from build123d import *

# Parameters (mm, degrees)
EXTRUDE1_DEPTH     = 16.75
SKETCH3_R          = 1.1
CUT_EXTRUDE1_DEPTH = 20.798295381
SKETCH5_R          = 4.1
CUT_EXTRUDE2_DEPTH = 24


with BuildPart() as part:
    # Sketch1 → Extrude1 (new body)
    with BuildSketch(Plane.XY):
        with BuildLine():
            Line((-4.6, -8.312039461), (-4.6, 8.312039461))
            ThreePointArc((-4.6, 8.312039461), (0, 9.5), (4.6, 8.312039461))
            Line((4.6, 8.312039461), (4.6, -8.312039461))
            ThreePointArc((4.6, -8.312039461), (0, -9.5), (-4.6, -8.312039461))
        make_face()
    extrude(amount=EXTRUDE1_DEPTH)

    # Sketch3 → Cut-Extrude1 (cut, through all)
    with BuildSketch(Plane.XY.offset(16.75)):
        with Locations((0, 6.715)):
            Circle(SKETCH3_R)
        with Locations(Location((0, -6.715, 0), (0, 0, 180))):
            Circle(SKETCH3_R)
    extrude(amount=-CUT_EXTRUDE1_DEPTH, mode=Mode.SUBTRACT)

    # Sketch5 → Cut-Extrude2 (cut)
    with BuildSketch(Plane(origin=(0, 0, 0), x_dir=(-1, 0, 0), z_dir=(0, 0, -1))):
        Circle(SKETCH5_R)
    extrude(amount=-CUT_EXTRUDE2_DEPTH, mode=Mode.SUBTRACT)


solid = part.part
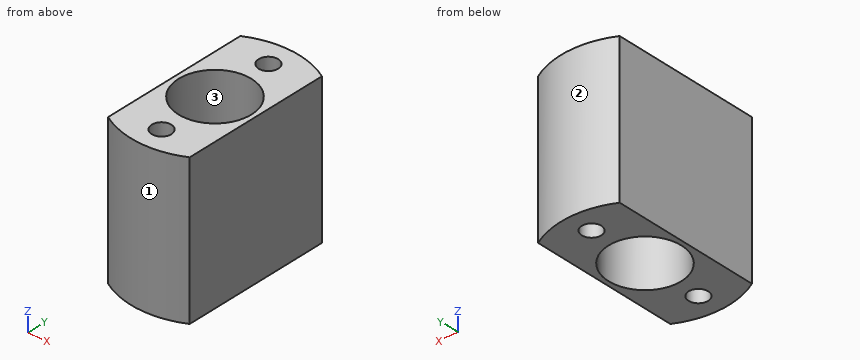
Can you work these out from the model? Positions are in its coordinate system, mm. Face numbers are marked on the shaded views. Coordinates: 2 decimals unless noted, no trailing zeros. Order: outer loops, then holes, each group sorted by start corner. A loop starts at its lowest first (then second) coordinate and runs counter-clockwise, first axis right, second up. Notation, with made-up numbers: M 88.25,-7.75 L 102.25,-7.75 A18 ccw 102.25,17.25 Z; hole C -24,76 d8. An arc over 180 degrees is marked long. Answer as CSV lines item,"result".
(1) Suppose I cut it at D-D on z = 11.5. Please give me the cut outline in (x, y) (3 decimals), plus the area to 3 significant figures.
Geometry check:
outline,"M -4.6,-8.312 A9.5 ccw 4.6,-8.312 L 4.6,8.312 A9.5 ccw -4.6,8.312 Z; hole C 0,0 d8.2; hole C 0,-6.715 d2.2; hole C 0,6.715 d2.2"
area,"107 mm^2"
(2) Suppose I cut it at B-B on x = 0. Please give me the cut outline in (y, z) (3 decimals).
Geometry check:
outline,"M -9.5,0 L -7.815,0 L -7.815,16.75 L -9.5,16.75 Z; M -5.615,0 L -4.1,0 L -4.1,16.75 L -5.615,16.75 Z; M 4.1,0 L 5.615,0 L 5.615,16.75 L 4.1,16.75 Z; M 7.815,0 L 9.5,0 L 9.5,16.75 L 7.815,16.75 Z"
(3) Suppose I cut it at A-A on y = 0. Please give me the cut outline in (x, z), plus the area to 4 significant figures.
Geometry check:
outline,"M -4.6,0 L -4.1,0 L -4.1,16.75 L -4.6,16.75 Z; M 4.1,0 L 4.6,0 L 4.6,16.75 L 4.1,16.75 Z"
area,"16.75 mm^2"
(4) If we mould it in two halves opening along Y, with no side actions, what happens to the marked faces 1, 2 and 3? For each: released by +Y, released by -Y, zero draft, split by the parting line, or undercut.
Geometry check:
face 1,"released by -Y"
face 2,"released by +Y"
face 3,"undercut"
(5) Please list where these lines run through material, in increasing order: L1, parallel to Y at x = 1.25, z = 15.25; L2, parallel to X at y = -2, z = 14.5; L3, parallel to X at y = -6, z = 8.5.
Geometry check:
L1,"-9.42 to -3.9, 3.9 to 9.42"
L2,"-4.6 to -3.58, 3.58 to 4.6"
L3,"-4.6 to -0.84, 0.84 to 4.6"
(6) Suppose I cut it at C-C on x = 1.5. Please give me the cut outline in (y, z).
Geometry check:
outline,"M -9.38,0 L -3.82,0 L -3.82,16.75 L -9.38,16.75 Z; M 3.82,0 L 9.38,0 L 9.38,16.75 L 3.82,16.75 Z"
